from build123d import *

# Parameters (mm, degrees)
F0_R     = 47.25
F1_DEPTH = 18
F2_R     = 15.75
F3_DEPTH = 5


with BuildPart() as f1:
    # F0 (on Top) → F1 (new body)
    with BuildSketch(Plane.XY):
        Circle(F0_R)
        with BuildLine():
            ThreePointArc((5, 42.9600104749), (30.5823682863, 30.5823682863), (42.9600104749, 5))
            ThreePointArc((42.9600104749, 5), (43.1774417551, 2.5042011663), (43.25, 0))
            ThreePointArc((43.25, 0), (43.1774417551, -2.5042011663), (42.9600104749, -5))
            ThreePointArc((42.9600104749, -5), (30.5823682863, -30.5823682863), (5, -42.9600104749))
            ThreePointArc((5, -42.9600104749), (0, -43.25), (-5, -42.9600104749))
            ThreePointArc((-5, -42.9600104749), (-30.5823682863, -30.5823682863), (-42.9600104749, -5))
            ThreePointArc((-42.9600104749, -5), (-43.25, 0), (-42.9600104749, 5))
            ThreePointArc((-42.9600104749, 5), (-30.5823682863, 30.5823682863), (-5, 42.9600104749))
            ThreePointArc((-5, 42.9600104749), (0, 43.25), (5, 42.9600104749))
        make_face(mode=Mode.SUBTRACT)
        with BuildLine():
            Line((42.9600104749, 5), (14.9352770312, 5))
            ThreePointArc((14.9352770312, 5), (15.4509075243, 3.0548251464), (15.7143044619, 1.0597807685))
            ThreePointArc((15.7143044619, 1.0597807685), (19.5862208579, 3.4586799782), (22.55, 0))
            ThreePointArc((22.55, 0), (19.5862208579, -3.4586799782), (15.7143044619, -1.0597807685))
            ThreePointArc((15.7143044619, -1.0597807685), (15.4509075243, -3.0548251464), (14.9352770312, -5))
            Line((14.9352770312, -5), (42.9600104749, -5))
            ThreePointArc((42.9600104749, -5), (43.1774417551, -2.5042011663), (43.25, 0))
            ThreePointArc((43.25, 0), (43.1774417551, 2.5042011663), (42.9600104749, 5))
        make_face()
        with BuildLine():
            ThreePointArc((-15.7143044619, 1.0597807685), (-15.4509075243, 3.0548251464), (-14.9352770312, 5))
            Line((-14.9352770312, 5), (-42.9600104749, 5))
            ThreePointArc((-42.9600104749, 5), (-43.25, 0), (-42.9600104749, -5))
            Line((-42.9600104749, -5), (-14.9352770312, -5))
            ThreePointArc((-14.9352770312, -5), (-15.4509075243, -3.0548251464), (-15.7143044619, -1.0597807685))
            ThreePointArc((-15.7143044619, -1.0597807685), (-22.55, 0), (-15.7143044619, 1.0597807685))
        make_face()
        with BuildLine():
            ThreePointArc((1.0597807685, 15.7143044619), (3.0548251464, 15.4509075243), (5, 14.9352770312))
            Line((5, 14.9352770312), (5, 42.9600104749))
            ThreePointArc((5, 42.9600104749), (0, 43.25), (-5, 42.9600104749))
            Line((-5, 42.9600104749), (-5, 14.9352770312))
            ThreePointArc((-5, 14.9352770312), (-3.0548251464, 15.4509075243), (-1.0597807685, 15.7143044619))
            ThreePointArc((-1.0597807685, 15.7143044619), (-2.0664906617, 21.8748214713), (3.5, 19.05))
            ThreePointArc((3.5, 19.05), (2.8248214713, 16.9835093383), (1.0597807685, 15.7143044619))
        make_face()
        with BuildLine():
            Line((5, -42.9600104749), (5, -14.9352770312))
            ThreePointArc((5, -14.9352770312), (3.0548251464, -15.4509075243), (1.0597807685, -15.7143044619))
            ThreePointArc((1.0597807685, -15.7143044619), (2.8248214713, -16.9835093383), (3.5, -19.05))
            ThreePointArc((3.5, -19.05), (-2.0664906617, -21.8748214713), (-1.0597807685, -15.7143044619))
            ThreePointArc((-1.0597807685, -15.7143044619), (-3.0548251464, -15.4509075243), (-5, -14.9352770312))
            Line((-5, -14.9352770312), (-5, -42.9600104749))
            ThreePointArc((-5, -42.9600104749), (0, -43.25), (5, -42.9600104749))
        make_face()
        with BuildLine():
            Line((-5, -14.9352770312), (-5, -11.7287041057))
            ThreePointArc((-5, -11.7287041057), (-9.0156114601, -9.0156114601), (-11.7287041057, -5))
            Line((-11.7287041057, -5), (-14.9352770312, -5))
            ThreePointArc((-14.9352770312, -5), (-11.1369318037, -11.1369318037), (-5, -14.9352770312))
        make_face()
        with BuildLine():
            Line((14.9352770312, -5), (11.7287041057, -5))
            ThreePointArc((11.7287041057, -5), (9.0156114601, -9.0156114601), (5, -11.7287041057))
            Line((5, -11.7287041057), (5, -14.9352770312))
            ThreePointArc((5, -14.9352770312), (11.1369318037, -11.1369318037), (14.9352770312, -5))
        make_face()
        with BuildLine():
            ThreePointArc((5, 11.7287041057), (9.0156114601, 9.0156114601), (11.7287041057, 5))
            Line((11.7287041057, 5), (14.9352770312, 5))
            ThreePointArc((14.9352770312, 5), (11.1369318037, 11.1369318037), (5, 14.9352770312))
            Line((5, 14.9352770312), (5, 11.7287041057))
        make_face()
        with BuildLine():
            ThreePointArc((-11.7287041057, 5), (-9.0156114601, 9.0156114601), (-5, 11.7287041057))
            Line((-5, 11.7287041057), (-5, 14.9352770312))
            ThreePointArc((-5, 14.9352770312), (-11.1369318037, 11.1369318037), (-14.9352770312, 5))
            Line((-14.9352770312, 5), (-11.7287041057, 5))
        make_face()
        with BuildLine():
            ThreePointArc((-5, 11.7287041057), (0, 12.75), (5, 11.7287041057))
            Line((5, 11.7287041057), (5, 14.9352770312))
            ThreePointArc((5, 14.9352770312), (3.0548251464, 15.4509075243), (1.0597807685, 15.7143044619))
            ThreePointArc((1.0597807685, 15.7143044619), (0, 15.55), (-1.0597807685, 15.7143044619))
            ThreePointArc((-1.0597807685, 15.7143044619), (-3.0548251464, 15.4509075243), (-5, 14.9352770312))
            Line((-5, 14.9352770312), (-5, 11.7287041057))
        make_face()
        with BuildLine():
            ThreePointArc((11.7287041057, 5), (12.4920670297, 2.5516193536), (12.75, 0))
            ThreePointArc((12.75, 0), (12.4920670297, -2.5516193536), (11.7287041057, -5))
            Line((11.7287041057, -5), (14.9352770312, -5))
            ThreePointArc((14.9352770312, -5), (15.4509075243, -3.0548251464), (15.7143044619, -1.0597807685))
            ThreePointArc((15.7143044619, -1.0597807685), (15.55, 0), (15.7143044619, 1.0597807685))
            ThreePointArc((15.7143044619, 1.0597807685), (15.4509075243, 3.0548251464), (14.9352770312, 5))
            Line((14.9352770312, 5), (11.7287041057, 5))
        make_face()
        with BuildLine():
            ThreePointArc((-11.7287041057, -5), (-12.75, 0), (-11.7287041057, 5))
            Line((-11.7287041057, 5), (-14.9352770312, 5))
            ThreePointArc((-14.9352770312, 5), (-15.4509075243, 3.0548251464), (-15.7143044619, 1.0597807685))
            ThreePointArc((-15.7143044619, 1.0597807685), (-15.5913200218, 0.5362208579), (-15.55, 0))
            ThreePointArc((-15.55, 0), (-15.5913200218, -0.5362208579), (-15.7143044619, -1.0597807685))
            ThreePointArc((-15.7143044619, -1.0597807685), (-15.4509075243, -3.0548251464), (-14.9352770312, -5))
            Line((-14.9352770312, -5), (-11.7287041057, -5))
        make_face()
        with BuildLine():
            Line((5, -14.9352770312), (5, -11.7287041057))
            ThreePointArc((5, -11.7287041057), (0, -12.75), (-5, -11.7287041057))
            Line((-5, -11.7287041057), (-5, -14.9352770312))
            ThreePointArc((-5, -14.9352770312), (-3.0548251464, -15.4509075243), (-1.0597807685, -15.7143044619))
            ThreePointArc((-1.0597807685, -15.7143044619), (0, -15.55), (1.0597807685, -15.7143044619))
            ThreePointArc((1.0597807685, -15.7143044619), (3.0548251464, -15.4509075243), (5, -14.9352770312))
        make_face()
    extrude(amount=F1_DEPTH)

    # F2 (on face) → F3 (join)
    with BuildSketch(Plane.XY.offset(18)):
        Circle(F2_R)
    extrude(amount=-F3_DEPTH)


solid = f1.part
Input: part model. Units: mm. Frame: model coordinates. A direction names the side the tool comes from. Coordinates: 2 decimals unless noted, no trailing zeros. Order: outer loops, then holes, each group sorted by start corner. A loop starts at its lowest first (then second) coordinate and runs counter-clockwise, first axis right, second up. Notation, with made-up numbers: M -23,-35.75 L 10,-35.75 A32 ccw 10,-0.75 Z; hole C 42.5,68 d8. An arc over 180 degrees is marked long. Answer in a Markdown table with one row per item.
(1) Draft query along X for faces 4 (the cylindrical face through (15.75, -0.01, 15.54)), 5 (the cylindrical face through (-37.496, -28.751, 8.874)), 6 (the flat face through (0, 0, 18)). Return one class per face: pulls with the +X half, pulls with the -X half, needs draft (parallel to the pull), parting line crosses it, or undercut.
Numbers:
| item | result |
|---|---|
| face 4 | undercut |
| face 5 | parting line crosses it |
| face 6 | needs draft |
(2) Access query for faces 1 (the flat face through (0, -14, 0)), 2 (the flat face through (0, 0, 13)), 3 (the flat face through (29, -5, 9)). Directions: +Z, -Z, +X, -X, +Y, -Y. A direction counts if a zero-diameter tool reaches every point of the face in a straight line with its end or side. Return the directions, or none.
Numbers:
| item | result |
|---|---|
| face 1 | -Z, +X, -X, +Y, -Y |
| face 2 | -Z |
| face 3 | +Z, -Z |
(3) Contact query for flat-ended pins moving along their axis: pin 1 Ø6 at (y, z) = (7, 8.5) entering from +X; pin 2 Ø6.5 at (x, y) = (0, -19.05) entering from -Z; pin 3 Ø5.5 at (x, z) = (-30.5, 6) entering from -Y; pin 4 Ø10 at (x, z) = (-34.5, 3) entering from -Y. Output: stop coordinate, or through.
Numbers:
| item | result |
|---|---|
| pin 1 | stops at x = 47.08 |
| pin 2 | passes through |
| pin 3 | stops at y = -38.24 |
| pin 4 | stops at y = -36.91 |
(4) Material intervals for line 1 (Y direction, x = 0, z = 10.75); line 2 (Y direction, x = -19.05, z = 12.5); line 3 (Y direction, x = -28, z = 11), sorted ascending. Write a range as [from, to].
Numbers:
| item | result |
|---|---|
| line 1 | y = [-47.25, -22.55], [-15.55, -12.75], [12.75, 15.55], [22.55, 47.25] |
| line 2 | y = [-43.24, -38.83], [-5, -3.5], [3.5, 5], [38.83, 43.24] |
| line 3 | y = [-38.06, -32.96], [-5, 5], [32.96, 38.06] |
(5) Section query A-A, the plane y = 35.5. Output: boundary loops of the cut face in (x, z), plus the area to 3 significant figures.
Numbers:
| item | result |
|---|---|
| outline | M -31.18,0 L -24.7,0 L -24.7,18 L -31.18,18 Z; M -5,0 L 5,0 L 5,18 L -5,18 Z; M 24.7,0 L 31.18,0 L 31.18,18 L 24.7,18 Z |
| area | 413 mm^2 |
(6) Section query B-B, the plane x = -20. Output: boundary loops of the cut face in (y, z).
Numbers:
| item | result |
|---|---|
| outline | M -42.81,0 L -38.35,0 L -38.35,18 L -42.81,18 Z; M -5,0 L -3.37,0 L -3.37,18 L -5,18 Z; M 3.37,0 L 5,0 L 5,18 L 3.37,18 Z; M 38.35,0 L 42.81,0 L 42.81,18 L 38.35,18 Z |
(7) Section query D-D, the plane x = 32. Output: boundary loops of the cut face in (y, z), plus the area to 3 significant figures.
Numbers:
| item | result |
|---|---|
| outline | M -34.76,0 L -29.1,0 L -29.1,18 L -34.76,18 Z; M -5,0 L 5,0 L 5,18 L -5,18 Z; M 29.1,0 L 34.76,0 L 34.76,18 L 29.1,18 Z |
| area | 384 mm^2 |
(8) Section query C-C, the plane y = 21. Output: boundary loops of the cut face in (x, z).
Numbers:
| item | result |
|---|---|
| outline | M -42.33,0 L -37.81,0 L -37.81,18 L -42.33,18 Z; M -5,0 L -2.91,0 L -2.91,18 L -5,18 Z; M 2.91,0 L 5,0 L 5,18 L 2.91,18 Z; M 37.81,0 L 42.33,0 L 42.33,18 L 37.81,18 Z |
